Geometry: final body of the model. Coordinates: model frame, mm. A direction names the side the tool comes from. Coordinates: 2 decimals unless noted, no trailing zeros. Order: outer loops, then holes, each group sorted by start corner. A loop starts at its lowest first (then second) coordinate and runs counter-clockwise, first axis right, second up. Notation, with made-up numbers: M -28,20.5 L 12,20.5 A31 ccw 12,50.5 Z; hole C -21.5,42 d6. An arc over 180 degrees is marked long. Write item = value, one per line.
from build123d import *

# Parameters (mm, degrees)
F0_W         = 304.8
F0_H         = 304.8
F1_DEPTH     = 3
F2_W         = 304.8
F2_H         = 304.8
F3_DEPTH     = 25.4
F4_T         = -2.54
F5_W         = 25.4
F5_H         = 25.4
F6_DEPTH     = 76.2
F7_T         = 2.54
F7_T3_DEPTH  = 30.48
F7_T5_DEPTH  = 30.48
F7_T7_DEPTH  = 30.94
F7_T9_DEPTH  = 304.8
F7_T11_DEPTH = 279.4
F7_T13_DEPTH = 279.4
F7_T15_DEPTH = 304.8
F8_W         = 25.4
F8_H         = 25.4
F8_W_2       = 20.32
F8_H_2       = 20.32
F9_DEPTH     = 76.2
F10_W        = 25.4
F10_H        = 50.8
F10_R        = 6.3459053742
F11_DEPTH    = 2.54
F12_W        = 25.4
F12_H        = 50.8
F12_R        = 6.35
F13_DEPTH    = 2.54
F14_W        = 25.4
F14_H        = 50.8
F14_R        = 6.35
F15_DEPTH    = 2.54
F16_W        = 25.4
F16_H        = 50.8
F16_R        = 6.35
F17_DEPTH    = 2.54


# Not quite as in the source:
# - a shell that OpenCascade refuses in one call is made with other operations: the cavity is built on its own and cut out


with BuildPart() as f1:
    # F0 (on Top) → F1 (new body)
    with BuildSketch(Plane.XY):
        with Locations((152.4, -152.4)):
            Rectangle(F0_W, F0_H)
    extrude(amount=F1_DEPTH)

    # F2 (on face) → F3 (join)
    with BuildSketch(Plane(origin=(0, 0, 0), x_dir=(1, 0, 0), z_dir=(0, 0, -1))):
        with Locations((152.4, 152.4)):
            Rectangle(F2_W, F2_H)
    extrude(amount=F3_DEPTH)

    # F4
    f4_openings = [f1.faces().sort_by_distance(p)[0] for p in [
        (152.4, -152.4, -25.4),
    ]]
    offset(amount=F4_T, openings=f4_openings)

    # F5 (on face) → F6 (join)
    with BuildSketch(Plane(origin=(0, 0, 0.46), x_dir=(1, 0, 0), z_dir=(0, 0, -1))):
        with Locations((289.56, 289.56)):
            Rectangle(F5_W, F5_H)
    extrude(amount=F6_DEPTH)

    # F7: shell of thickness 2.54, made by hand


with BuildPart() as f7_core1:
    # F7_t2: copy of F1
    add(f1.part)

    # the walls: a layer under each face that stays
    f7_faces = [f7_core1.faces().sort_by_distance(p)[0] for p in [
        (152.4, -304.8, -11.2),
        (152.4, -152.4, 3),
        (304.8, -152.4, -11.2),
        (2.38125, -120.4148148148, -25.4),
        (0, -152.4, -11.2),
        (152.4, 0, -11.2),
        (2.54, -152.4, -12.47),
        (289.56, -302.26, -50.57),
        (139.7, -302.26, -12.47),
        (302.26, -139.7, -12.47),
        (302.26, -289.56, -50.57),
        (152.4, -2.54, -12.47),
        (152.4, -152.4, 0.46),
        (276.86, -289.56, -37.64),
        (289.56, -276.86, -37.64),
    ]]
    thicken(f7_faces, amount=-F7_T, mode=Mode.SUBTRACT)

    # F7_s4 → F7_t3 (cut)
    with BuildSketch(Plane.YZ.offset(274.32)):
        Polygon((-302.2854, -25.4254), (-302.26, -22.86), (-299.72, -22.86), (-299.72, -25.4), align=None)
        Polygon((-276.8346, 0.4346), (-276.86, 3), (-279.4, 3), (-279.4, 0.46), align=None)
    extrude(amount=F7_T3_DEPTH, mode=Mode.SUBTRACT)

    # F7_s6 → F7_t5 (cut)
    with BuildSketch(Plane.XZ.offset(274.32)):
        Polygon((302.2854, -25.4254), (302.26, -22.86), (299.72, -22.86), (299.72, -25.4), align=None)
        Polygon((276.8346, 0.4346), (276.86, 3), (279.4, 3), (279.4, 0.46), align=None)
    extrude(amount=F7_T5_DEPTH, mode=Mode.SUBTRACT)

    # F7_s8 → F7_t7 (cut)
    with BuildSketch(Plane.XY.offset(-27.94)):
        Polygon((2.5654, -2.5654), (0, -2.54), (0, 0), (2.54, 0), align=None)
        Polygon((2.5654, -302.2346), (0, -302.26), (0, -304.8), (2.54, -304.8), align=None)
        Polygon((276.8346, -302.2346), (276.86, -304.8), (279.4, -304.8), (279.4, -302.26), align=None)
        Polygon((302.2346, -2.5654), (304.8, -2.54), (304.8, 0), (302.26, 0), align=None)
        Polygon((302.2346, -276.8346), (304.8, -276.86), (304.8, -279.4), (302.26, -279.4), align=None)
    extrude(amount=F7_T7_DEPTH, mode=Mode.SUBTRACT)

    # F7_s10 → F7_t9 (cut)
    with BuildSketch(Plane.XZ):
        Polygon((2.5654, 0.4346), (0, 0.46), (0, 3), (2.54, 3), align=None)
    extrude(amount=F7_T9_DEPTH, mode=Mode.SUBTRACT)

    # F7_s12 → F7_t11 (cut)
    with BuildSketch(Plane.YZ):
        Polygon((-302.2346, 0.4346), (-304.8, 0.46), (-304.8, 3), (-302.26, 3), align=None)
    extrude(amount=F7_T11_DEPTH, mode=Mode.SUBTRACT)

    # F7_s14 → F7_t13 (cut)
    with BuildSketch(Plane.XZ):
        Polygon((302.2346, 0.4346), (304.8, 0.46), (304.8, 3), (302.26, 3), align=None)
    extrude(amount=F7_T13_DEPTH, mode=Mode.SUBTRACT)

    # F7_s16 → F7_t15 (cut)
    with BuildSketch(Plane.YZ):
        Polygon((-2.5654, 0.4346), (0, 0.46), (0, 3), (-2.54, 3), align=None)
    extrude(amount=F7_T15_DEPTH, mode=Mode.SUBTRACT)


with BuildPart() as f1_1:
    add(f1.part)

    # what is left inside the walls is the cavity
    f7_cavity = [f7_core1.part.solids().sort_by_distance(p)[0] for p in [
        (290.83, -279.4254, -50.34),
    ]]
    add(f7_cavity, mode=Mode.SUBTRACT)

    # F8 (on face) → F9 (join)
    with BuildSketch(Plane(origin=(0, 0, 0.46), x_dir=(1, 0, 0), z_dir=(0, 0, -1))):
        with Locations((15.24, 15.24)):
            Rectangle(F8_W, F8_H)
        with Locations((15.24, 15.24)):
            Rectangle(F8_W_2, F8_H_2, mode=Mode.SUBTRACT)
        with Locations((289.56, 15.24)):
            Rectangle(F8_W, F8_H)
        Polygon((279.4, 5.08), (279.4, 15.24), (279.4, 25.4), (299.72, 25.4), (299.72, 5.08), align=None, mode=Mode.SUBTRACT)
        with Locations((15.24, 289.56)):
            Rectangle(F8_W, F8_H)
        Polygon((25.4, 279.4), (15.24, 279.4), (5.08, 279.4), (5.08, 299.72), (25.4, 299.72), align=None, mode=Mode.SUBTRACT)
    extrude(amount=F9_DEPTH)

    # F10 (on face) → F11 (join)
    with BuildSketch(Plane(origin=(0, 0, -75.74), x_dir=(1, 0, 0), z_dir=(0, 0, -1))):
        with Locations((289.56, 2.54)):
            Rectangle(F10_W, F10_H)
        with Locations((289.56, -10.1621253416)):
            Circle(F10_R, mode=Mode.SUBTRACT)
    extrude(amount=F11_DEPTH)

    # F12 (on face) → F13 (join)
    with BuildSketch(Plane(origin=(0, 0, -75.74), x_dir=(1, 0, 0), z_dir=(0, 0, -1))):
        with Locations((15.24, 2.54)):
            Rectangle(F12_W, F12_H)
        with Locations((15.24, -10.16)):
            Circle(F12_R, mode=Mode.SUBTRACT)
    extrude(amount=F13_DEPTH)

    # F14 (on face) → F15 (join)
    with BuildSketch(Plane(origin=(0, 0, -75.74), x_dir=(1, 0, 0), z_dir=(0, 0, -1))):
        with Locations((15.24, 302.26)):
            Rectangle(F14_W, F14_H)
        with Locations((15.24, 314.96)):
            Circle(F14_R, mode=Mode.SUBTRACT)
    extrude(amount=F15_DEPTH)

    # F16 (on face) → F17 (join)
    with BuildSketch(Plane(origin=(0, 0, -75.74), x_dir=(1, 0, 0), z_dir=(0, 0, -1))):
        with Locations((289.56, 302.26)):
            Rectangle(F16_W, F16_H)
        with Locations((289.56, 314.96)):
            Circle(F16_R, mode=Mode.SUBTRACT)
    extrude(amount=F17_DEPTH)


solid = f1_1.part
1) Pin query (flat end, axial travel): pin 1 (7.5 mm diameter, centred on x = 18.5, z = -39, fed in from -Y); pin 2 (12.5 mm diameter, centred on x = 15, y = -315, fed in from +Z); pin 3 (1 mm diameter, centred on y = -281, z = -63.5, fed in from -X). Return the tip coordinate at first contact, or that it passes through.
Numbers:
pin_1 = -302.26
pin_2 = -75.74
pin_3 = 2.54
2) Line query: L1, parallel to Y at x = 15.24, z = -77; L2, parallel to X at y = 10.16, z = -77.1; L3, parallel to X at y = -288.5, z = -9. Output: solid intervals per line, ascending.
Numbers:
L1 = -327.66 to -321.31, -308.61 to -276.86, -27.94 to 3.81, 16.51 to 22.86
L2 = 2.54 to 8.89, 21.59 to 27.94, 276.86 to 283.21, 295.91 to 302.26
L3 = 0 to 5.08, 25.4 to 27.94, 276.86 to 279.4, 302.26 to 304.8
3) Section A-A, the plane x = 289.56. Give the number of separate pieces and of enclosed holes in the cut face, and give its area (3 significant figures).
Numbers:
separate_pieces = 3
enclosed_holes = 2
area = 1,810 mm²
4) Mould query, pull axis Z, two halves, no side actions, for faces 1 (the face through (302.26, -13, -51)), 2 (the face through (289, -3, -78.28)), 3 (the face through (15, -5.08, -37)). Classes: pulls with the +Z half, pulls with the -Z half, needs draft (parallel to the pull), parting line crosses it, or undercut.
Numbers:
face_1 = needs draft
face_2 = pulls with the -Z half
face_3 = undercut
5) Section C-C, the plane y = -314.96. Return loops of the section in (x, z).
Numbers:
outline = M 2.54,-78.28 L 8.89,-78.28 L 8.89,-75.74 L 2.54,-75.74 Z; M 21.59,-78.28 L 27.94,-78.28 L 27.94,-75.74 L 21.59,-75.74 Z; M 276.86,-78.28 L 283.21,-78.28 L 283.21,-75.74 L 276.86,-75.74 Z; M 295.91,-78.28 L 302.26,-78.28 L 302.26,-75.74 L 295.91,-75.74 Z
6) Set-up query: faces 4 (the face through (150, -304.8, -11)), 5 (the face through (27.94, -291, -38)), 6 (the face through (15, -2.54, -50)), 7 (the face through (15, -279.4, -37)), 8 (the face through (12, -321, -75.74)). Return all of +Z, -Z, +X, -X, +Y, -Y with unobstructed straight access to the full face (end or side cutting, diameter ignored); none if empty.
Numbers:
face_4 = +Z, +X, -X, -Y
face_5 = -Z
face_6 = +X, -X, +Y
face_7 = none
face_8 = +X, -X, -Y
